Input: part model. Units: mm. Frame: model coordinates. A direction names the side the tool comes from. Round coordinates to 2 decimals unless told otherwise and drop trailing zeros. Loops run counter-clockwise (first coordinate to the right, second up) from the corner with the lowest first, then second, coordinate; pieces in that order, holes last. Notation, with made-up numbers: M 63.25,-38.75 L 112.25,-38.75 A8 ccw 112.25,-32.75 Z; hole C -27,48.25 d8. An arc over 180 degrees is marked long. Return JSON: item names as keys, results as strings. Group by question number.
1) Section C-C (y = -13.75). Output: boundary loops of the cut face in (x, z), plus the area to 3 significant figures.
2) Section A-A (x = 0). Output: boundary loops of the cut face in (y, z).
3) Contact query for flat-ended pins moving along their axis: P1, Ø4, axis at x = 1.5, z = 3.5, coming from the +Y side; P2, Ø1, axis at x = 3, z = -2.5, coming from the +Y side; P3, Ø1, axis at x = -3, y = -14, coming from the +Z side. Output: stop coordinate, or through.
4) Material intervals for line 1 (Y direction, x = 1.5, z = -1.5); line 2 (Y direction, x = -1.75, z = -3.75); line 3 (Y direction, x = 0.75, z = -3), sorted ascending. Write a range as from..to.
5) Mould query, pull axis Y, two halves, no side actions, for faces 3 (the face through (-1, -15.5, 2)), 4 (the face through (0.77, -14.76, 1.85)), 5 (the face through (0, -25.5, 0)), 6 (the face through (-3.04, -13.01, -3.32)). Classes: +Y half, -Y half, draft (parallel to the pull), parting line (faces both ways), or undercut.
6) Access query for faces 1 (the face through (4, -12, 0)), 2 (the face through (-0.1, -20.3, -2.5)). Directions: +Z, -Z, +X, -X, +Y, -Y. A direction counts if a zero-diameter tool reaches every point of the face in a straight line with its end or side. Return the directions, or none.
7) Section B-B (y = -21). Output: boundary loops of the cut face in (x, z).
from build123d import *

# Parameters (mm, degrees)
CHANFREIN1_SIZE = 0.5
CONG_1_R        = 1


with BuildPart() as part:
    # Esquisse2 → Base-Révolution (revolve)
    with BuildSketch(Plane.XY, mode=Mode.PRIVATE) as base_r_volution_sk:
        with BuildLine():
            Line((1.5, -7.5), (2.85, -12))
            Line((2.85, -12), (4.5, -12))
            Line((4.5, -12), (4.5, -14))
            Line((4.5, -14), (2.5, -14))
            Line((2.5, -14), (2.002434927, -14))
            Line((2.002434927, -14), (2.002434927, -15.5))
            Line((2.002434927, -15.5), (2.5, -15.5))
            Line((2.5, -15.5), (2.5, -25.5))
            Line((2.5, -25.5), (0, -25.5))
            Line((0, -25.5), (0, 0))
            ThreePointArc((0, 0), (3.824264635, -3.135147073), (1.5, -7.5))
        make_face()
    revolve(base_r_volution_sk.sketch.rotate(Axis((0, 10.187617919, 0), (0, -1, 0)), 90), axis=Axis((0, 10.187617919, 0), (0, -1, 0)))  # turned: the seam where the file's is

    # Chanfrein1
    chanfrein1_edges = [part.edges().sort_by_distance(p)[0] for p in [
        (0, -25.5, -2.5),
    ]]
    chamfer(chanfrein1_edges, length=CHANFREIN1_SIZE)

    # Congé1
    cong_1_edges = [part.edges().sort_by_distance(p)[0] for p in [
        (0, -12, -2.85),
    ]]
    fillet(cong_1_edges, radius=CONG_1_R)


solid = part.part
Returned:
{
 "1": {"outline": "C 0,0 d9", "area": "63.6 mm^2"},
 "2": {"outline": "M -25.5,-2 L -25,-2.5 L -15.5,-2.5 L -15.5,-2 L -14,-2 L -14,-4.5 L -12,-4.5 L -12,-3.59 A1 cw -11.29,-2.64 L -7.5,-1.5 A3.9 ccw long -7.5,1.5 L -11.29,2.64 A1 cw -12,3.59 L -12,4.5 L -14,4.5 L -14,2 L -15.5,2 L -15.5,2.5 L -25,2.5 L -25.5,2 Z"},
 "3": {"P1": "stops at y = -0.44", "P2": "stops at y = -2", "P3": "stops at z = 3.74"},
 "4": {"line 1": "y = -25.38..-15.5, -14..-9.57, -7.17..-0.63", "line 2": "y = -14..-12", "line 3": "y = -14..-11.87, -6.28..-1.52"},
 "5": {"face 3": "undercut", "face 4": "undercut", "face 5": "-Y half", "face 6": "draft"},
 "6": {"face 1": "none", "face 2": "-Y"},
 "7": {"outline": "C 0,0 d5"}
}
